Can you work these out from the drawing? Everything is in mm from the part's minimum corner. A direction names the side the tool comes from. Round coordinates to 2 decimals unless told otherwise and drop trailing zeros. Write each loop counter-clockwise with the first axis right and the second up, starting at its lowest first coordinate (ties: lowest second). Pieces come first, ordered by that corner, then holes. Notation, with made-up numbers: (61, -24) -> (72, -24) arc R35 cw to (72, 13) -> close; hole circle Ø6 at (46, 34.5). An arc over 180 degrees is marked (long way). One line per question, with ' | ' between items. Start each with the question number.
1. Imagine slicing it at D-D, the plane z = 0.25. List the corners of the cut face in (x, y) for me, and give its area (3 significant figures).
2. For pin 1 Ø1.5 at (x, y) = (1.5, 7) entering from +Z; pin 2 Ø0.7 at (y, z) = (9.5, 1.5) entering from +X; pin 3 Ø0.7 at (x, y) = (1.5, 9) entering from +Z; pin 4 Ø0.7 at (x, y) = (1.5, 8) entering from -Z, each with a flat end and sliding along its axis, tell me the tip position at first contact or that it passes through.
3. Imagine slicing it at C-C, the plane x = 0.2. List the corners of the cut face in (y, z) for me, and give its area (3 significant figures).
4. Imagine slicing it at B-B, the plane y = 5.5. List the corners of the cut face in (x, z) for me.
5. Imagine slicing it at A-A, the plane z = 1.25. List the corners of the cut face in (x, y) for me.
6. If I drill on line 1 along X through (y, z) = (2, 1.05); line 2 along Y through (x, z) = (0.5, 0.9), over which ranges is the centre line in solid material (lowest first)? Write a range as [from, to].
7. For the marked faces 1, 2 and 3, which set-ups out of +Z, -Z, +X, -X, +Y, -Y let a thin tool reach every point of the face, with its end or its side?
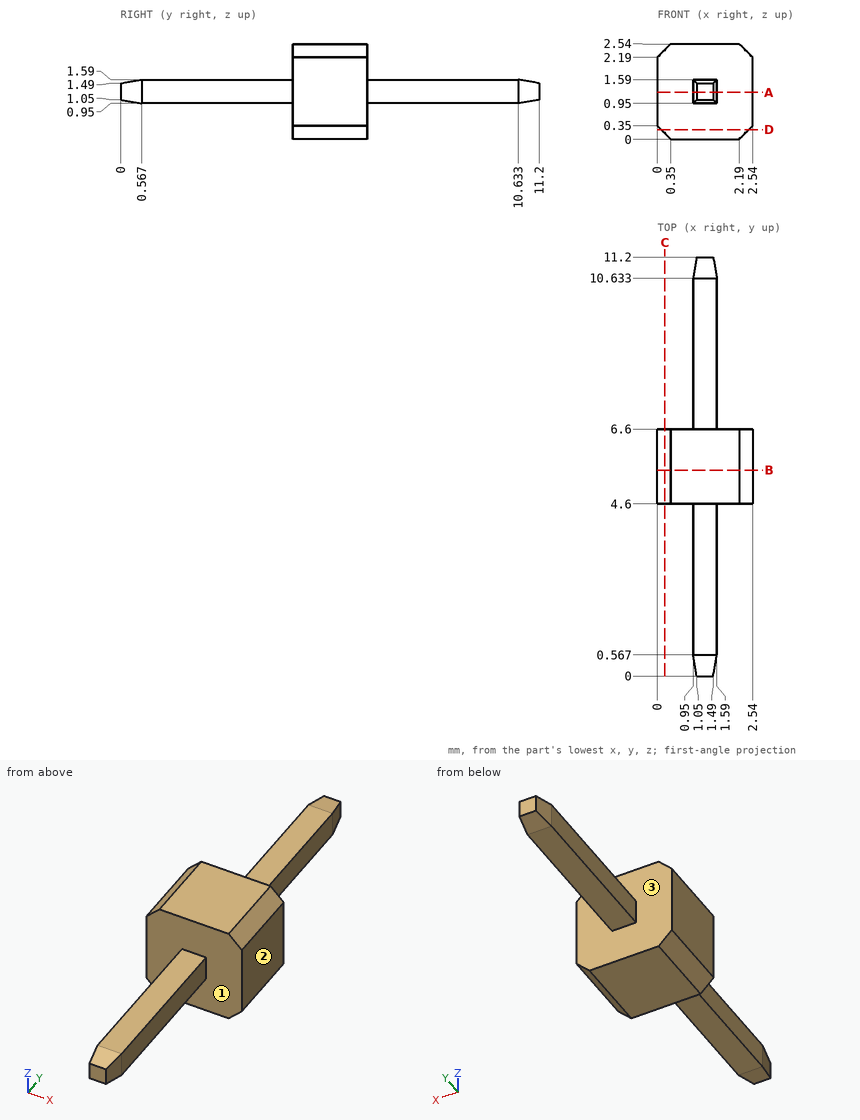
Geometry results:
1) outline: (0.1, 4.6) -> (2.44, 4.6) -> (2.44, 6.6) -> (0.1, 6.6) -> close | area: 4.68 mm2
2) pin 1: stops at z = 2.54 | pin 2: stops at x = 1.59 | pin 3: stops at z = 1.59 | pin 4: stops at z = 0.95
3) outline: (4.6, 0.15) -> (6.6, 0.15) -> (6.6, 2.39) -> (4.6, 2.39) -> close | area: 4.48 mm2
4) outline: (0, 0.35) -> (0.35, 0) -> (2.19, 0) -> (2.54, 0.35) -> (2.54, 2.19) -> (2.19, 2.54) -> (0.35, 2.54) -> (0, 2.19) -> close
5) outline: (0, 4.6) -> (0.95, 4.6) -> (0.95, 0.57) -> (1.05, 0) -> (1.49, 0) -> (1.59, 0.57) -> (1.59, 4.6) -> (2.54, 4.6) -> (2.54, 6.6) -> (1.59, 6.6) -> (1.59, 10.63) -> (1.49, 11.2) -> (1.05, 11.2) -> (0.95, 10.63) -> (0.95, 6.6) -> (0, 6.6) -> close
6) line 1: x = [0.95, 1.59] | line 2: y = [4.6, 6.6]
7) face 1: -Y | face 2: +Z, -Z, +X, +Y, -Y | face 3: +Y
